CAD build for the part. Positions are in the model's coordinates, mm. A direction names the side the tool comes from. Give positions to 0.01 mm unless a question says otherwise; leave off trailing zeros. Order: outer loops, then holes, each group sorted by start corner. A loop starts at its lowest first (then second) coordinate and runs counter-clockwise, first axis right, second up.
Item 1: Band-saw the part on A-A on z = -2.25. Give the cut face in (x, y).
Item 2: Flat gauge pins, fed straight in: P1, Ø2, axis at x = 5, z = -5.5, coming from the -Y side; P2, Ø2, axis at x = 6.5, y = 5.5, coming from the +Z side; P3, Ø2, axis at x = 3.5, z = -1.5, coming from the +Y side; P4, Ø0.9, axis at x = 3, y = 1.5, coming from the -Z side. Where does each tip first touch, or does it go through?
Item 3: Band-saw the part on D-D on z = -10.5. Give the cut face in (x, y) (3 decimals), plus the area to 3 significant figures.
Item 4: Which spindle directions (+Z, -Z, +X, -X, +Y, -Y) get a long thin tool onto all of the face, cutting with end or side? Do faces 4 (the flat face through (5.525, 5, -10)), 5 (the flat face through (4, 0, -7)), 6 (the flat face through (4, 1, -13)), 7 (the cylindrical face through (4, 1.5, -9.9)), 8 (the flat face through (0, 4, -7)). Say none if no direction does.
Item 5: Two-plate mould, pull along X, no slides. Class faces 1 (the flat face through (3.98, 3.92, -9.31)), 2 (the flat face through (4, 3, -1)), 3 (the flat face through (8, 4, -7)): released by +X, released by -X, zero draft, split by the parting line, or undercut.
Item 6: Band-saw the part on C-C on y = 1. Give the cut face in (x, z), plus the area to 3 significant figures.
Item 7: Band-saw the part on B-B on x = 6.25. Give the cut face in (y, z).
Item 8: Wall check: L1, parallel to X at y = 2.35, z = -10.75; L2, parallel to X at y = 2.25, z = -12.5 (3 decimals); L3, parallel to Z at x = 4.5, y = 2.5. Give the ranges that are in metal, low to high.
```python
from build123d import *

# Parameters (mm, degrees)
SKETCH_6_W          = 8
SKETCH_6_H          = 13
SKETCH_6_R          = 0.85
EXTRUDE_1_DEPTH     = 3
EXTRUDE_2_DEPTH     = 8
SKETCH_9_W          = 3.05
SKETCH_9_H          = 3.05
CUT_EXTRUDE_3_DEPTH = 19.796569864


with BuildPart() as part:
    # 草图6 → 凸台-拉伸1 (new body)
    with BuildSketch(Plane(origin=(0, 0, 0), x_dir=(1, 0, 0), z_dir=(0, 1, 0))):
        with Locations((4, 6.5)):
            Rectangle(SKETCH_6_W, SKETCH_6_H)
        with Locations(Location((4, 2.25, 0), (0, 0, 270))):
            Circle(SKETCH_6_R, mode=Mode.SUBTRACT)
        with Locations(Location((4, 10.75, 0), (0, 0, 90))):
            Circle(SKETCH_6_R, mode=Mode.SUBTRACT)
    extrude(amount=EXTRUDE_1_DEPTH)

    # 草图8 → 凸台-拉伸2 (add)
    with BuildSketch(Plane(origin=(8, 0, 0), x_dir=(0, 0, -1), z_dir=(1, 0, 0))):
        Polygon((13, 3), (14.75, 6.031088913), (8, 9.92820323), (4, 3), align=None)
    extrude(amount=-EXTRUDE_2_DEPTH)

    # 草图9 → 切除-拉伸3 (cut, through all)
    with BuildSketch(Plane(origin=(0, -0.982050808, -1.700961894), x_dir=(1, 0, 0), z_dir=(0, 0.500000000000004, 0.8660254037844364))):
        with Locations((4, 9.573076211)):
            Rectangle(SKETCH_9_W, SKETCH_9_H)
    extrude(amount=-CUT_EXTRUDE_3_DEPTH, mode=Mode.SUBTRACT)


solid = part.part
```
The answers:
1. outline: (0, 0) - (3.15, 0) - (3.15, 3) - (0, 3) - close; (4.85, 0) - (8, 0) - (8, 3) - (4.85, 3) - close
2. P1: stops at y = 0
2. P2: stops at z = -4.87
2. P3: stops at y = 3
2. P4: stops at z = -13
3. outline: (0, 0) - (3.188, 0) - (3.188, 3) - (4.812, 3) - (4.812, 0) - (8, 0) - (8, 8.485) - (0, 8.485) - close; hole (2.475, 3.231) - (5.525, 3.231) - (5.525, 6.753) - (2.475, 6.753) - close
3. area: 52.3 mm2
4. face 4: none
4. face 5: +Z, -Z, +X, -X, -Y
4. face 6: -Z, +X, -X, -Y
4. face 7: -Y
4. face 8: +Z, -Z, -X, +Y, -Y
5. face 1: undercut
5. face 2: zero draft
5. face 3: released by +X
6. outline: (0, -13) - (8, -13) - (8, 0) - (0, 0) - close; hole circle Ø1.7 at (4, -10.75); hole circle Ø1.7 at (4, -2.25)
6. area: 99.5 mm2
7. outline: (0, -13) - (3, -13) - (6.03, -14.75) - (9.93, -8) - (3, -4) - (3, 0) - (0, 0) - close
8. L1: x = 0 to 3.15, 4.85 to 8
8. L2: x = 0 to 2.475, 5.525 to 8
8. L3: z = -11.77 to -11.44, -10.06 to -2.94, -1.56 to 0
